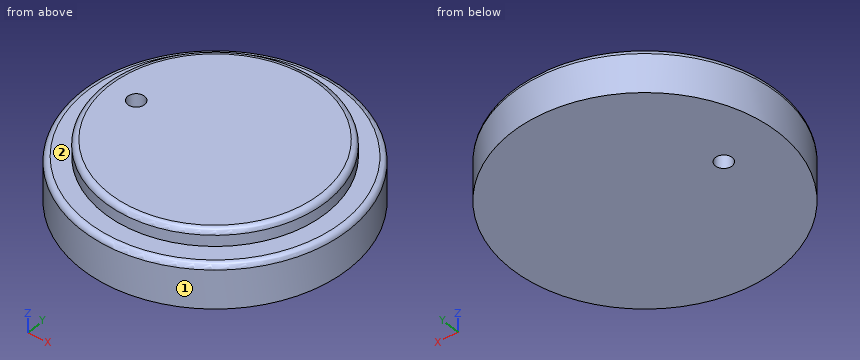
```python
from build123d import *

# Parameters (mm, degrees)
F0_R     = 76.2
F1_DEPTH = 25.4
F2_R     = 63.5
F3_DEPTH = 9.53262
F4_R     = 3.175
F6_D     = 9.525


with BuildPart() as f1:
    # F0 (on Top) → F1 (new body)
    with BuildSketch(Plane.XY):
        Circle(F0_R)
    extrude(amount=F1_DEPTH)

    # F2 (on face) → F3 (join)
    with BuildSketch(Plane.XY.offset(25.4)):
        Circle(F2_R)
    extrude(amount=F3_DEPTH)

    # F4
    f4_edges = [f1.edges().sort_by_distance(p)[0] for p in [
        (-76.2, 0, 25.4),
        (-63.5, 0, 34.93262),
    ]]
    fillet(f4_edges, radius=F4_R)

    # F6 (through all)
    with Locations(Plane.XY.offset(34.93262)):
        with Locations((-44.45, 0)):
            Hole(F6_D / 2)


solid = f1.part
```
Part model, mm, in its own coordinate system. Face numbers are marked on the shaded views. A direction names the side the tool comes from. Round coordinates to 2 decimals unless told otherwise and drop trailing zeros. Write each loop counter-clockwise with the first axis right and the second up, starting at its lowest first coordinate (ties: lowest second). Pieces come first, ordered by that corner, then holes.
Item 1: Probe L1, parallel to Z at x = 16, y = 69; L2, parallel to Y at x = -44.45, z = 9; L3, parallel to Y at x = -42.5, z = 9. List the from-to ranges inside material, lowest first.
Results:
L1: z = 0 to 25.4
L2: y = -61.89 to -4.76, 4.76 to 61.89
L3: y = -63.25 to -4.34, 4.34 to 63.25
Item 2: Which spindle directions (+Z, -Z, +X, -X, +Y, -Y) get a long thin tool onto all of the face, cutting with end or side? Do the marked faces 1 and 2. Say none if no direction does.
Results:
face 1: +Z, -Z
face 2: +Z
Item 3: Drop flat-ended pins along their axis: pin 1 Ø5 at (y, z) = (-50.5, 30.5) entering from -X; pin 2 Ø2 at (x, z) = (-16.5, 8) entering from -Y; pin 3 Ø3 at (y, z) = (-45.5, 30.5) entering from +X. Give the stop position or say it passes through.
Results:
pin 1: stops at x = -41.57
pin 2: stops at y = -74.61
pin 3: stops at x = 45.78
Item 4: Cut at B-B, the plane x = 0. Give the cut face in (y, z) (3 decimals).
Results:
outline: (-76.2, 0) - (76.2, 0) - (76.2, 22.225) arc R3.175 ccw to (73.025, 25.4) - (63.5, 25.4) - (63.5, 31.758) arc R3.175 ccw to (60.325, 34.933) - (-60.325, 34.933) arc R3.175 ccw to (-63.5, 31.758) - (-63.5, 25.4) - (-73.025, 25.4) arc R3.175 ccw to (-76.2, 22.225) - close
